Read the model definition and answer for the solid it produces. Units are mm, in the model's axes. A direction names the side the tool comes from. Coordinates: 2 decimals unless noted, no trailing zeros. Put each result on its own line as item: value.
Autodesk Inventor part; units mm, degrees
ref_plane "YZ Plane" through (0, 0, 0) normal (1, 0, 0) x (0, 1, 0)
ref_plane "XZ Plane" through (0, 0, 0) normal (0, 1, 0) x (-1, 0, 0)
ref_plane "XY Plane" through (0, 0, 0) normal (0, 0, 1) x (1, 0, 0)
sketch "Sketch1" plane through (0, 0, 0) normal (0, 0, 1) x (1, 0, 0)
  line L0 (-36.9502, 25.0692) -> (31.8498, 25.0692)
  line L1 (31.8498, 25.0692) -> (31.8498, -108.9308)
  line L2 (31.8498, -108.9308) -> (-36.9502, -108.9308)
  line L3 (-36.9502, -108.9308) -> (-36.9502, 25.0692)
  point P0 (0, 0)
  dimension "d0" = 68.8
  dimension "d1" = 134
extrude "Extrusion1" add sketch "Sketch1" along normal blind 9.3
sketch "Sketch2" plane through (0, 0, 9.3) normal (0, 0, 1) x (1, 0, 0)
  line L0 (-33.5502, 9.0692) -> (28.4498, 9.0692)
  line L1 (28.4498, 9.0692) -> (28.4498, -92.4308)
  line L2 (28.4498, -92.4308) -> (-33.5502, -92.4308)
  line L3 (-33.5502, -92.4308) -> (-33.5502, 9.0692)
  line L4 (-36.9502, 25.0692) -> (-36.9502, -108.9308)
  line L5 (31.8498, 25.0692) -> (-36.9502, 25.0692)
  line L6 (-36.9502, -108.9308) -> (31.8498, -108.9308)
  point P0 (0, 0)
  dimension "d4" = 62
  dimension "d5" = 3.4
  dimension "d6" = 16
  dimension "d7" = 16.5
extrude "Extrusion2" cut sketch "Sketch2" against normal blind 0.1
sketch "Sketch3" plane through (-36.9502, -108.9308, 0) normal (0, -1, 0) x (1, 0, 0)
  line L0 (30.8, 5.2565) -> (38, 5.2565)
  line L1 (38, 5.2565) -> (38, 3.1565)
  line L2 (38, 3.1565) -> (30.8, 3.1565)
  line L3 (30.8, 3.1565) -> (30.8, 5.2565)
  line L4 (0, 0) -> (0, 9.3)
  point P0 (36.9502, 0)
  dimension "d10" = 7.2
  dimension "d11" = 2.1
  dimension "d12" = 30.8
extrude "Extrusion3" cut sketch "Sketch3" against normal blind 5
fillet "Fillet1" radius 5 4 edges at (31.8498, -108.9308, 4.65) (-36.9502, -108.9308, 4.65) (31.8498, 25.0692, 4.65) (-36.9502, 25.0692, 4.65)
fillet "Fillet2" radius 0.5 16 edges at (30.3853, -107.4663, 9.3) (31.8498, -41.9308, 9.3) (30.3853, 23.6048, 9.3) (-2.5502, 25.0692, 9.3) (-35.4858, 23.6048, 9.3) (-36.9502, -41.9308, 9.3) (-35.4858, -107.4663, 9.3) (-2.5502, -108.9308, 9.3) (30.3853, -107.4663, 0) (-2.5502, -108.9308, 0) (-35.4858, -107.4663, 0) (-36.9502, -41.9308, 0) (-35.4858, 23.6048, 0) (-2.5502, 25.0692, 0) (30.3853, 23.6048, 0) (31.8498, -41.9308, 0)
properties part number "Nexus4"
Q1. For a pull along X with two mould halves and no side action, classify faces 1 (the face through (30.35, -107.5, 4.71)), 2 (the face through (-35, -42, 9.3)), 3 (the face through (-2, -106, 3.156)) as +X half, -X half, draft (parallel to the pull), parting line (faces both ways), or undercut.
Answers below:
face 1: +X half
face 2: draft
face 3: undercut
Q2. Given pin 1 (2.5 mm diameter, centred on y = -106, z = 4.5, fed in from -X); pin 2 (1 mm diameter, centred on y = -105.5, z = 4.5, fed in from +X), each flat-ended and moving along its own axis, determine where each tip first touches the part or whether it passes through.
Answers below:
pin 1: stops at x = -36.88
pin 2: stops at x = 31.73
Q3. A tool of negligible diameter and unlimited length cuts with its end or side. For faces 4 (the face through (-3, -106, 5.256)), 5 (the face through (-3, 25.069, 5)), 6 (the face through (-3, -41, 9.2)), from which of +Z, -Z, +X, -X, +Y, -Y can it reach the whole face along a straight path? Write none if from no direction.
Answers below:
face 4: -Y
face 5: +Z, -Z, +X, -X, +Y
face 6: +Z
Q4. Consider line 1 along Z through (x, y) = (-14, -35); line 2 along Y through (x, z) = (27, 6); line 3 along Y through (x, z) = (28, 5.75). Determine where each line is inside the solid, lowest interval first.
Answers below:
line 1: z = 0 to 9.2
line 2: y = -108.93 to 25.07
line 3: y = -108.8 to 24.94
